Check sheet for the drawn part. Datum: minimum x, y, z corner. Units: mm. A direction names the side the tool comes from. Round coordinates to 2 decimals unless told otherwise and drop trailing zeros. Loops run counter-clockwise (first coordinate to the right, second up) from the corner with the lowest first, then second, coordinate; pieces in that order, holes last.
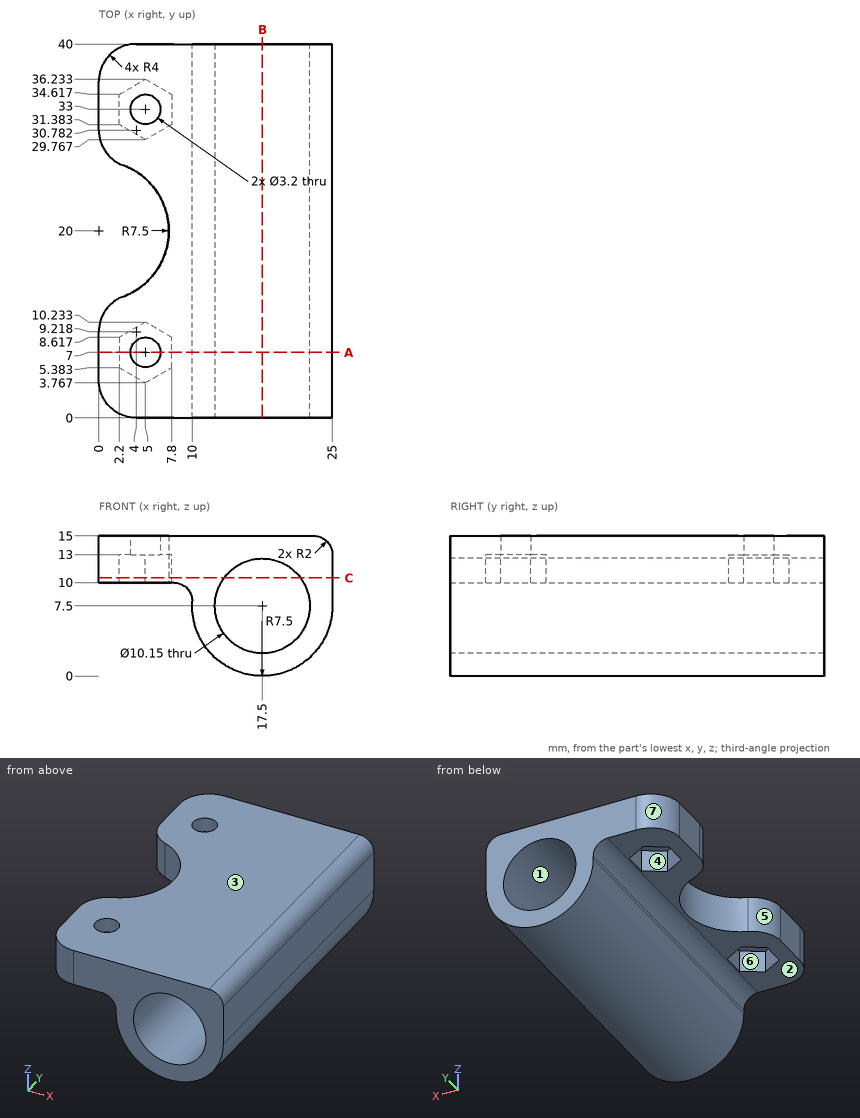
1. Section check B-B (x = 17.5). Enter the section's corners in (y, z) (1 decimal).
2. Section check C-C (z = 10.5). Enter the section's corners in (x, y), then the cut area to 3 significant figures.
3. Section check A-A (y = 7). Give the number of separate pieces and of enclosed holes in the cut face, then the cut area to 3 significant figures.
4. Tool access check on the marked faces 5, 6 and 7. Record the directions out of +Z, -Z, +X, -X, +Y, -Y that give a thin tool (end or side, any length) a straight path to the whole face; none if there is none.
5. Gauge pin test, flat ends, axial feed: P1, Ø1.5, axis at x = 3, z = 9.5, coming from the -Y side (1 decimal); P2, Ø6, axis at x = 9.5, y = 20.5, coming from the -Z side; P3, Ø3, axis at x = 20, y = 11, coming from the -Z side. Record the tip position at first contact, or that the pin passes through.
6. Release check for a two-part mould opening along Z. For the marked faces 1, 2, 3 and 4 record: released by +Z, released by -Z, zero draft, split by the parting line, or undercut.
7. Scan lines: L1, parallel to Y at x = 5, z = 14.4; L2, parallel to X at y = 9.5, z = 11.5 (1 decimal); L3, parallel to X at y = 8, z = 7.5 (1 decimal). Record each from-to range of solid material in increasing order.
Taken from the geometry:
1. outline: (0, 0) - (40, 0) - (40, 2.4) - (0, 2.4) - close; (0, 12.6) - (40, 12.6) - (40, 15) - (0, 15) - close
2. outline: (0, 4) arc R4 ccw to (4, 0) - (13.41, 0) - (13.41, 40) - (4, 40) arc R4 ccw to (0, 36) - (0, 30.78) arc R4 ccw to (2.61, 27.03) arc R7.5 cw to (2.61, 12.97) arc R4 ccw to (0, 9.22) - close; (21.59, 0) - (25, 0) - (25, 40) - (21.59, 40) - close; hole (2.2, 5.38) - (5, 3.77) - (7.8, 5.38) - (7.8, 8.62) - (5, 10.23) - (2.2, 8.62) - close; hole (2.2, 31.38) - (5, 29.77) - (7.8, 31.38) - (7.8, 34.62) - (5, 36.23) - (2.2, 34.62) - close
2. area: 519 mm2
3. separate pieces: 2
3. enclosed holes: 1
3. area: 147 mm2
4. face 5: +Z, -Z, -X
4. face 6: -Z
4. face 7: +Z, -Z, -X, +Y
5. P1: stops at y = 0
5. P2: stops at z = 1.91
5. P3: stops at z = 0.07
6. face 1: undercut
6. face 2: released by -Z
6. face 3: released by +Z
6. face 4: zero draft
7. L1: y = 0 to 5.4, 8.6 to 14.41, 25.59 to 31.4, 34.6 to 40
7. L2: x = 0 to 3.7, 6.3 to 14.4, 20.6 to 25
7. L3: x = 10 to 12.4, 22.6 to 25
